Model file for the job. Use its own axes, mm. Face numbers are marked on the shaded views. A direction names the side the tool comes from. Coordinates: 2 decimals unless noted, no trailing zeros. Order: outer loops, then holes, each group sorted by start corner. A loop starts at its lowest first (then second) coordinate and runs counter-clockwise, first axis right, second up. Notation, with made-up numbers: (20.5, -11.5) -> (46.5, -11.5) arc R25 cw to (46.5, 4.5) -> close; hole circle Ø2 at (-19.5, 69.5). An arc over 180 degrees is marked (long way). Return JSON: item names as keys, results as strings. Group by question number.
1) Which spindle directions (+Z, -Z, +X, -X, +Y, -Y) get a long thin tool onto all of the face, cutting with end or side? Do the marked faces 5, 6 and 7. Say none if no direction does.
2) Cut at D-D (z = -8.5). Write the cut outline in (x, y), and give its area (3 significant figures).
3) Cut at A-A (x = 0). Write the cut outline in (y, z).
4) Probe line 1 (X direction, y = 1.5, z = 19); line 2 (X direction, y = 42, z = -11); line 3 (Z direction, x = 20.5, y = 6.5). List the from-to ranges inside material, lowest first.
5) Flat gauge pins, fed straight in: pin 1 (2 mm diameter, centred on x = 29.5, z = 25, fed in from -Y); pin 2 (8 mm diameter, centred on x = -32.5, y = 62.5, fed in from -Z); pin 3 (9 mm diameter, centred on x = 0, y = 72, fed in from -Z); pin 4 (11.5 mm diameter, centred on x = -19.05, y = 61, fed in from +Z). Where does each tip first touch, or does it go through?
6) Cut at B-B (y = 72). Write the cut outline in (x, z).
7) Pull direction Y, two halves, no side cores. Call the marked faces 1, 2, 3 and 4: +Y half, -Y half, draft (parallel to the pull), parting line (faces both ways), or undercut.
8) Cut at C-C (x = 41). Write the cut outline in (y, z), and give its area (3 significant figures).
Autodesk Fusion 360 part; units mm, degrees
sketch "Sketch1" plane through (0, 0, 0) normal (0, 0, 1) x (1, 0, 0)
  circle A0 centre (-41, 0) radius 5
  line L0 (-32, 50) -> (-32, 0)
  line L1 (32, 50) -> (32, 0)
  arc A1 (-32, 38.4187) -> (32, 38.4187) centre (0, 0) ccw
  arc A2 (-32, 25.632) -> (32, 25.632) centre (0, 0) ccw construction
  arc A3 (-32, 0) -> (32, 0) centre (0, 0) ccw
  arc A4 (32, 50) -> (-32, 50) centre (0, 50) ccw
  circle A5 centre (0, 50) radius 22 construction
  circle A6 centre (0, 72) radius 5
  line L2 (6, 50) -> (6, 0)
  line L3 (-6, 50) -> (-6, 0)
  arc A7 (-6, 0) -> (6, 0) centre (0, 0) ccw
  arc A8 (6, 50) -> (-6, 50) centre (0, 50) ccw
  line L4 (-32, 50) -> (-22, 50)
  line L5 (32, 50) -> (22, 50)
  line L6 (-22, 50) -> (-22, 0)
  line L7 (22, 50) -> (22, 0)
  arc A9 (-22, 0) -> (22, 0) centre (0, 0) ccw
  line L8 (-32, 12) -> (-22, 12)
  line L9 (22, 12) -> (32, 12)
  dimension "d1" = 100
  dimension "d2" = 82
  dimension "d3" = 10
  dimension "d4" = 41
  dimension "d5" = 64
  dimension "d6" = 64
  dimension "d7" = 50
  dimension "d8" = 50
  dimension "d9" = 12
  dimension "d10" = 12
  dimension "d11" = 44
  dimension "d12" = 44
  dimension "d13" = 10
  dimension "d14" = 22
  dimension "d15" = 12
  dimension "d16" = 12
extrude "Extrude1" add sketch "Sketch1" against normal blind 16 contours A0 | L0 L1 A1 A3 makes body 1
extrude "Extrude3" cut sketch "Sketch1" against normal blind 5 contours A0 | L0 L1 A1 A3 bodies 1
extrude "Extrude2" add sketch "Sketch1" against normal blind 16 separate body contours A4 L4 L5 L6 L7 A9 | A6 makes body 2
extrude "Extrude4" add sketch "Sketch1" along normal blind 40 and the other way up to surface (16 mm away) contours L0 L4 L6 L8 | L1 L5 L7 L9 | L0 L1 A3 L6 L7 A9 L8 L9 bodies 1 2
chamfer "Chamfer1" distance 40 angle 45 2 edges at (-27, 50, 40) (27, 50, 40) on bodies 1
extrude "Extrude6" cut sketch "Sketch1" against normal through all contours A0 bodies 1
extrude "Extrude7" cut sketch "Sketch1" against normal through all contours A6 bodies 1
pattern_circular "C-Pattern1" count 3 over 180 about axis through (0, 0, 1.75) along (0, 0, 1) of "Extrude6"
pattern_circular "C-Pattern2" count 3 over 120 about axis through (0, 50, 0) along (0, 0, -1) both ways of "Extrude7"
equation "d4 = d2 / 2"
equation "d14 = d11 / 2"
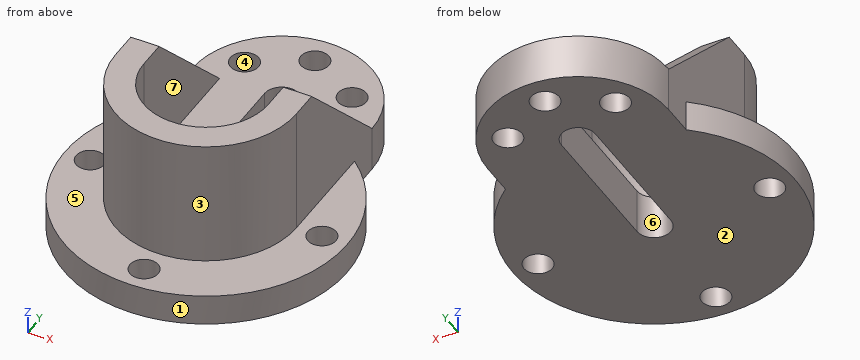
Answers below:
{
 "1": {"face 5": "+Z, -Y", "face 6": "+Z, -Z", "face 7": "+Z, +Y"},
 "2": {"outline": "(-32, 38.42) arc R50 ccw (long way) to (32, 38.42) -> (32, 50) arc R32 ccw to (-32, 50) -> close; hole circle Ø10 at (-41, 0); hole circle Ø10 at (-19.05, 61); hole (-6, 0) arc R6 ccw to (6, 0) -> (6, 50) arc R6 ccw to (-6, 50) -> close; hole circle Ø10 at (0, -41); hole circle Ø10 at (0, 72); hole circle Ø10 at (19.05, 61); hole circle Ø10 at (41, 0)", "area": "8,510 mm^2"},
 "3": {"outline": "(-50, -16) -> (-46, -16) -> (-46, -5) -> (-50, -5) -> close; (-36, -16) -> (-6, -16) -> (-6, 0) -> (-22, 0) -> (-22, 40) -> (-32, 40) -> (-32, -5) -> (-36, -5) -> close; (56, -16) -> (67, -16) -> (67, 0) -> (56, 0) -> close; (77, -16) -> (82, -16) -> (82, 0) -> (77, 0) -> close"},
 "4": {"line 1": "x = -32 to -22, 22 to 32", "line 2": "x = -32 to -6, 6 to 32", "line 3": "z = -16 to 0"},
 "5": {"pin 1": "stops at y = -14.55", "pin 2": "stops at z = -16", "pin 3": "passes through", "pin 4": "stops at z = 0"},
 "6": {"outline": "(-23.24, -16) -> (-5, -16) -> (-5, 0) -> (-23.24, 0) -> close; (5, -16) -> (23.24, -16) -> (23.24, 0) -> (5, 0) -> close"},
 "7": {"face 1": "parting line", "face 2": "draft", "face 3": "-Y half", "face 4": "undercut"},
 "8": {"outline": "(-28.62, -16) -> (-5, -16) -> (-5, -5) -> (-28.62, -5) -> close; (5, -16) -> (28.62, -16) -> (28.62, -5) -> (5, -5) -> close", "area": "520 mm^2"}
}
